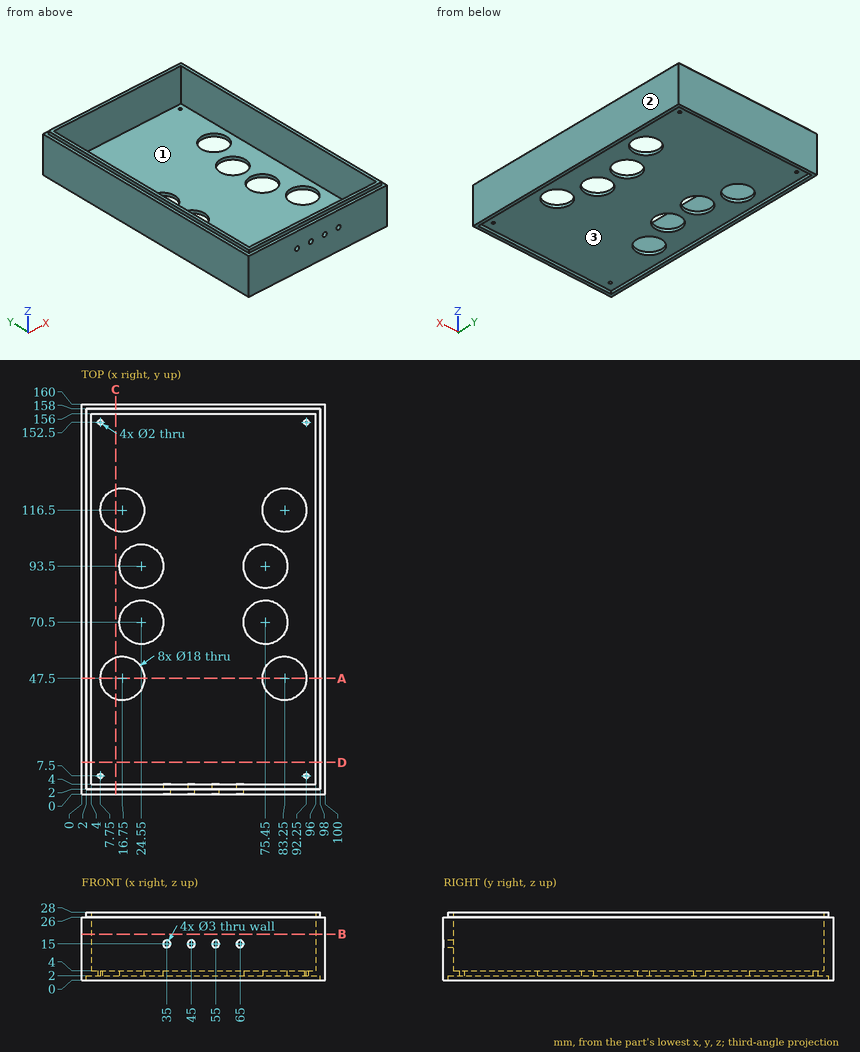
Design review of the part shown in the three views and the two pictorial views. Dimensions are in mm from the part's minimum x, y and z. A direction names the side the tool comes from. Round coordinates to 2 decimals unless told otherwise and drop trailing zeros. Write each loop counter-clockwise with the first axis right and the second up, starting at its lowest first coordinate (ties: lowest second). Pieces come first, ordered by that corner, then holes.
1) Take a section at C-C on x = 14. Give the boundary of the cut face in (y, z).
Answer below:
outline: (0, 0) - (2, 0) - (2, 2) - (38.93, 2) - (38.93, 4) - (4, 4) - (4, 28) - (2, 28) - (2, 26) - (0, 26) - close; (56.07, 2) - (107.93, 2) - (107.93, 4) - (56.07, 4) - close; (125.07, 2) - (158, 2) - (158, 0) - (160, 0) - (160, 26) - (158, 26) - (158, 28) - (156, 28) - (156, 4) - (125.07, 4) - close
2) Machinability: for the marked faces 1, 2 and 3, which of the approach directions +Z, -Z, +X, -X, +Y, -Y give a long, thin tool a straight path to every point of the face, cutting with its end or side? Answer none if there is none.
Answer below:
face 1: +Z
face 2: +Z, -Z, +X, +Y, -Y
face 3: -Z
3) Take a section at D-D on y = 13. Give the boundary of the cut face in (x, z).
Answer below:
outline: (0, 0) - (2, 0) - (2, 2) - (98, 2) - (98, 0) - (100, 0) - (100, 26) - (98, 26) - (98, 28) - (96, 28) - (96, 4) - (4, 4) - (4, 28) - (2, 28) - (2, 26) - (0, 26) - close
4) Insertion check: pin 1 Ø3 at (x, y) = (92.25, 152.5) entering from -Z; pin 2 Ø1 at (x, z) = (31, 27) entering from -Y; pin 3 Ø10 at (x, y) = (70, 137) entering from +Z. Each pin has a flat end and moves straight along its axis. Give the tip position at first contact, or say it passes through.
Answer below:
pin 1: stops at z = 2
pin 2: stops at y = 2
pin 3: stops at z = 4
5) Take a section at B-B on z = 19. Give the boundary of the cut face in (x, y).
Answer below:
outline: (0, 0) - (100, 0) - (100, 160) - (0, 160) - close; hole (4, 4) - (96, 4) - (96, 156) - (4, 156) - close
6) For line 1 along X through (y, z) = (7.5, 3); line 2 along X through (y, z) = (26, 9.25); line 3 along Y through (x, z) = (10, 17.5), list the stretches that pass through material, from the lowest coordinate up.
Answer below:
line 1: x = 0 to 6.75, 8.75 to 91.25, 93.25 to 100
line 2: x = 0 to 4, 96 to 100
line 3: y = 0 to 4, 156 to 160
7) Take a section at A-A on y = 47.5. Give the boundary of the cut face in (x, z), then the cut area to 3 significant figures.
Answer below:
outline: (0, 0) - (2, 0) - (2, 2) - (7.75, 2) - (7.75, 4) - (4, 4) - (4, 28) - (2, 28) - (2, 26) - (0, 26) - close; (25.75, 2) - (74.25, 2) - (74.25, 4) - (25.75, 4) - close; (92.25, 2) - (98, 2) - (98, 0) - (100, 0) - (100, 26) - (98, 26) - (98, 28) - (96, 28) - (96, 4) - (92.25, 4) - close
area: 320 mm2
